Could you check a few things on this drawing? It's one solid part, dimensions in mm from its lowest x, y, z. A direction names the side the tool comes from. Give positions to 0.01 mm unless a question says otherwise; leave off trailing zeros. Order: outer loops, then holes, each group sorted by start corner. A loop starts at its lowest first (then second) coordinate and runs counter-clockwise, first axis right, second up. Notation, with made-up numbers: M 53.5,-2 L 105.5,-2 A12 cw 105.5,17 Z; hole C 40.25,53.25 d9. An arc over 180 degrees is marked long. Use one line per item in the form item = value. Start each with the question number.
1. I need wall thicknesses on L1, parallel to X at y = 14.25, z = 19; L2, parallel to X at y = 20.25, z = 34. Which ranges of each line are inside material? Lowest first, please.
2. I want a section at D-D, the plane y = 18.25. List the corners of the cut face in (x, z) for me, and give its area (3 significant figures).
3. Will these pins go through, and if not, where does the flat tip stop? P1, Ø12, axis at x = 15, y = 16, coming from the +Z side; P2, Ø2, axis at x = 40, z = 25, coming from the -Y side; P3, Ø6.5, axis at y = 12.5, z = 22.5, coming from the +X side; P4, Ø0.6, axis at x = 40, y = 4, coming from the -Z side.
4. I want a section at C-C, the plane z = 34.5. List the corners of the cut face in (x, y) for me.
5. I want a section at A-A, the plane y = 5.25. List the corners of the cut face in (x, z) for me.
6. We'd pull the mould along X, two halves only. Please class the marked faces 1, 2, 3 and 4: +X half, -X half, draft (parallel to the pull), parting line (faces both ways), or undercut.
7. I want a section at B-B, the plane x = 32. List the corners of the cut face in (y, z) for me.
8. For the marked faces 5, 6 and 7, which set-ups out of +Z, -Z, +X, -X, +Y, -Y let a thin tool reach every point of the face, with its end or its side?
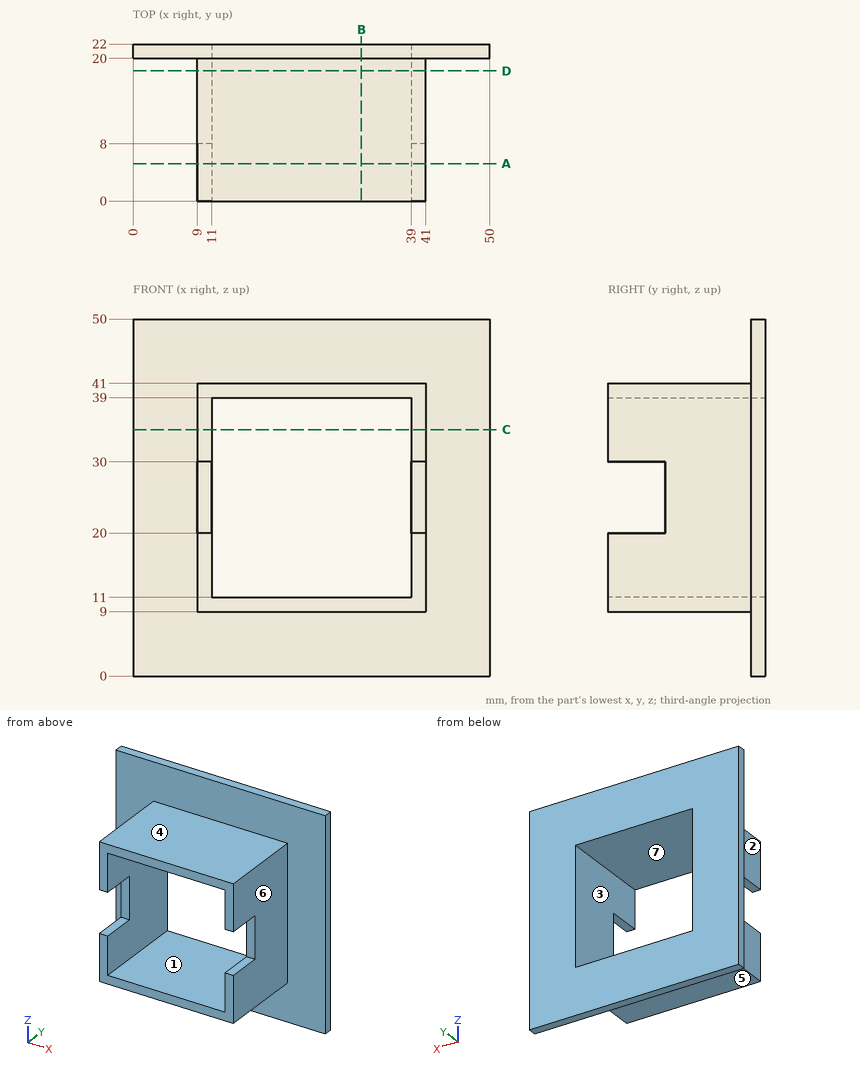
Check result:
q1.L1 = 9 to 11, 39 to 41
q1.L2 = 0 to 11, 39 to 50
q2.outline = M 9,9 L 41,9 L 41,41 L 9,41 Z; hole M 11,11 L 39,11 L 39,39 L 11,39 Z
q2.area = 240 mm2
q3.P1 = 50
q3.P2 = 8
q3.P3 = 41
q3.P4 = 9
q4.outline = M 0,20 L 9,20 L 9,0 L 11,0 L 11,22 L 0,22 Z; M 39,0 L 41,0 L 41,20 L 50,20 L 50,22 L 39,22 Z
q5.outline = M 9,9 L 41,9 L 41,20 L 39,20 L 39,11 L 11,11 L 11,20 L 9,20 Z; M 9,30 L 11,30 L 11,39 L 39,39 L 39,30 L 41,30 L 41,41 L 9,41 Z
q6.face_1 = undercut
q6.face_2 = -X half
q6.face_3 = undercut
q6.face_4 = draft
q7.outline = M 0,9 L 20,9 L 20,0 L 22,0 L 22,11 L 0,11 Z; M 0,39 L 22,39 L 22,50 L 20,50 L 20,41 L 0,41 Z
q8.face_5 = -Z, +X, -X, -Y
q8.face_6 = +Z, -Z, +X, -Y
q8.face_7 = +Y, -Y
